```python
from build123d import *

# Parameters (mm, degrees)
EXTRUDE_1_DEPTH          = 211
SHELL_2_T                = 10
CUT_EXTRUDE_2_DEPTH      = 306.363666708
CUT_EXTRUDE_2_DEPTH_BACK = 306.363666708
SKETCH_8_R               = 10
CUT_EXTRUDE_6_DEPTH      = 10
SKETCH_13_R              = 10
CUT_EXTRUDE_7_DEPTH      = 10


with BuildPart() as part:
    # 草图1 → 凸台-拉伸1 (new body)
    with BuildSketch(Plane(origin=(0, 0, 0), x_dir=(1, 0, 0), z_dir=(0, 1, 0))):
        Polygon((0, 152.5), (0, 0), (122, 0), (159.592352403, 65.111864338), (86.265, 152.5), align=None)
        Polygon((-122, 0), (0, 0), (0, 152.5), (-86.265, 152.5), (-159.592352403, 65.111864338), align=None)
    extrude(amount=EXTRUDE_1_DEPTH)

    # 抽壳2 (no face opened: a closed hollow body)
    add(offset(amount=-SHELL_2_T, mode=Mode.PRIVATE), mode=Mode.SUBTRACT)

    # 草图5 → 切除-拉伸-薄壁2 (cut, two sides)
    with BuildSketch(Plane(origin=(0, 0, 0), x_dir=(0, 0, -1), z_dir=(1, 0, 0))) as cut_extrude_2_sk:
        Polygon((79.3, 211), (65.111864338, 10), (0, 10), (0, 211), (10, 211), (10, 20), (55.792859546, 20), (69.32482043, 211.704125378), align=None)
    extrude(amount=CUT_EXTRUDE_2_DEPTH, mode=Mode.SUBTRACT)
    extrude(cut_extrude_2_sk.sketch, amount=-CUT_EXTRUDE_2_DEPTH_BACK, mode=Mode.SUBTRACT)


with BuildPart() as cut_extrude_2_kept_piece:
    # of the separate pieces the step leaves, the one the design keeps (cut_extrude_2_pieces_kept)
    add(part.part.solids().sort_by_distance((122, 0, 0))[0])

    # 草图8 → 切除-拉伸6 (cut)
    with BuildSketch(Plane(origin=(0, 211, 0), x_dir=(1, 0, 0), z_dir=(0, 1, 0))):
        with Locations(Location((-54.9, 115.9, 0), (0, 0, 270))):
            Circle(SKETCH_8_R)
        with Locations(Location((54.9, 115.9, 0), (0, 0, 90))):
            Circle(SKETCH_8_R)
    extrude(amount=-CUT_EXTRUDE_6_DEPTH, mode=Mode.SUBTRACT)

    # 草图13 → 切除-拉伸7 (cut)
    with BuildSketch(Plane(origin=(0, 10, 0), x_dir=(1, 0, 0), z_dir=(0, 1, 0))):
        with Locations(Location((-73.2, 30.5, 0), (0, 0, 270))):
            Circle(SKETCH_13_R)
        with Locations(Location((73.2, 30.5, 0), (0, 0, 90))):
            Circle(SKETCH_13_R)
    extrude(amount=-CUT_EXTRUDE_7_DEPTH, mode=Mode.SUBTRACT)


solid = cut_extrude_2_kept_piece.part
```
Geometry check sheet. Reference: the model listing, model coordinates, mm. A direction names the side the tool comes from. Coordinates: 2 decimals unless noted, no trailing zeros. Order: outer loops, then holes, each group sorted by start corner. A loop starts at its lowest first (then second) coordinate and runs counter-clockwise, first axis right, second up. Notation, with made-up numbers: (46, 17) - (67, 17) arc R26 ccw to (67, 33) - close; hole circle Ø10 at (0, 61.25). An arc over 180 degrees is marked (long way). Answer in a Markdown table with one row per item. Add a question column.
1. Draft check along Y on faces 1 (the face through (82.072, 5.07, -35.114)), 2 (the face through (-2, 0, -77)), 3 (the face through (-2, 10, -72)), 4 (the face through (-2, 211, -116)). Enter one of: +Y half, -Y half, draft (parallel to the pull), parting line (faces both ways), or undercut.
2. Access from +Z, -Z, +X, -X, +Y, -Y to the whole of each face (thin tool, end or side, straight path). Record for faces 5 (the face through (-0.74, 207.75, -79.07)), 6 (the face through (114.525, 104.163, -103.264)), 7 (the face through (58.73, 206.07, -125.137)).
3. Section check C-C (x = 26). Enter the section's corners in (y, z).
4. Section check D-D (z = -115.9). Enter the section's corners in (x, y), plus the area to 3 significant figures.
5. Material ranges on L1, parallel to X at y = 8, z = -30; L2, parallel to Y at x = -40.5, z = -115; L3, parallel to X at y = 205.5, z = -115.9, recorded low to high. Write a range as [from, to].
6. Section check B-B (z = -31.5). Enter the section's corners in (x, y), plus the area to 3 significant figures.
7. Gauge pin test, flat ends, axial feed: pin 1 Ø1 at (x, z) = (55, -78) entering from -Y; pin 2 Ø4 at (x, y) = (25.5, 119) entering from +Z; pin 3 Ø12 at (x, z) = (54.9, -115.9) entering from +Y; pin 4 Ø2 at (y, z) = (133, -116) entering from -X. Record the tip position at first contact, or that the pin passes through.
8. Section check A-A (x = -73.2). Enter the section's corners in (y, z), plus the area to 3 significant figures.
Data:
| question | item | result |
|---|---|---|
| 1 | face 1 | draft |
| 1 | face 2 | -Y half |
| 1 | face 3 | undercut |
| 1 | face 4 | +Y half |
| 2 | face 5 | +Z, +X, -X, +Y |
| 2 | face 6 | +Z |
| 2 | face 7 | +Y |
| 3 | outline | (0, -152.5) - (211, -152.5) - (211, -79.3) - (201, -78.59) - (201, -142.5) - (10, -142.5) - (10, 0) - (0, 0) - close |
| 4 | outline | (-116.98, 0) - (116.98, 0) - (116.98, 211) - (64.9, 211) - (64.9, 201) - (103.92, 201) - (103.92, 10) - (-103.92, 10) - (-103.92, 201) - (-64.9, 201) - (-64.9, 211) - (-116.98, 211) - close; (-44.9, 201) - (44.9, 201) - (44.9, 211) - (-44.9, 211) - close |
| 4 | area | 9,270 mm² |
| 5 | L1 | x = [-139.32, -83.19], [-63.21, 63.21], [83.19, 139.32] |
| 5 | L2 | y = [0, 10], [201, 211] |
| 5 | L3 | x = [-116.98, -64.9], [-44.9, 44.9], [64.9, 116.98] |
| 6 | outline | (-140.19, 0) - (-83.15, 0) - (-83.15, 10) - (-140.19, 10) - close; (-63.25, 0) - (63.25, 0) - (63.25, 10) - (-63.25, 10) - close; (83.15, 0) - (140.19, 0) - (140.19, 10) - (83.15, 10) - close |
| 6 | area | 2,410 mm² |
| 7 | pin 1 | stops at y = 0 |
| 7 | pin 2 | stops at z = -142.5 |
| 7 | pin 3 | stops at y = 10 |
| 7 | pin 4 | stops at x = -117.73 |
| 8 | outline | (0, -152.5) - (211, -152.5) - (211, -79.3) - (201, -78.59) - (201, -142.5) - (10, -142.5) - (10, -40.5) - (0, -40.5) - close; (0, -20.5) - (10, -20.5) - (10, 0) - (0, 0) - close |
| 8 | area | 3,970 mm² |
